Can you work these out from the model? Positions are in its coordinate system, mm. Face numbers are marked on the shaded views. A direction names the side the tool comes from. Give positions to 0.01 mm unless a question says otherwise; leave off trailing zeros. Order: outer loops, then holes, each group sorted by start corner. A loop starts at its lowest first (then second) coordinate and runs counter-clockwise, first axis right, second up. Notation, with made-up numbers: (82.5, 33.25) - (122.5, 33.25) arc R25 ccw to (122.5, 51.25) - close; hole circle Ø1 at (60.5, 37). An arc over 180 degrees is marked (long way). Answer as CSV lines item,"result".
```python
from build123d import *

# Parameters (mm, degrees)
SKETCH_1_W      = 120
SKETCH_1_H      = 150
EXTRUDE_1_DEPTH = 10
CHAMFER_1_SIZE  = 10
EXTRUDE_2_DEPTH = 20


with BuildPart() as part:
    # 草图1 → 凸台-拉伸1 (new, symmetric)
    with BuildSketch(Plane.XY):
        Rectangle(SKETCH_1_W, SKETCH_1_H)
    extrude(amount=EXTRUDE_1_DEPTH, both=True)

    # 倒角1
    chamfer_1_edges = [part.edges().sort_by_distance(p)[0] for p in [
        (-60, 75, 0),
        (60, 75, 0),
    ]]
    chamfer(chamfer_1_edges, length=CHAMFER_1_SIZE)

    # 草图2 → 凸台-拉伸2 (add)
    with BuildSketch(Plane(origin=(60, 0, 0), x_dir=(0, 0, -1), z_dir=(1, 0, 0))):
        Polygon((10, -75), (60, -75), (60, -65), (20, -15), (10, -15), align=None)
    extrude_2 = extrude(amount=-EXTRUDE_2_DEPTH)

    # 镜向1: 凸台-拉伸2 across plane
    add(extrude_2.mirror(Plane(origin=(0, 0, 0), x_dir=(0, 0, 1), z_dir=(1, 0, 0))))


solid = part.part
```
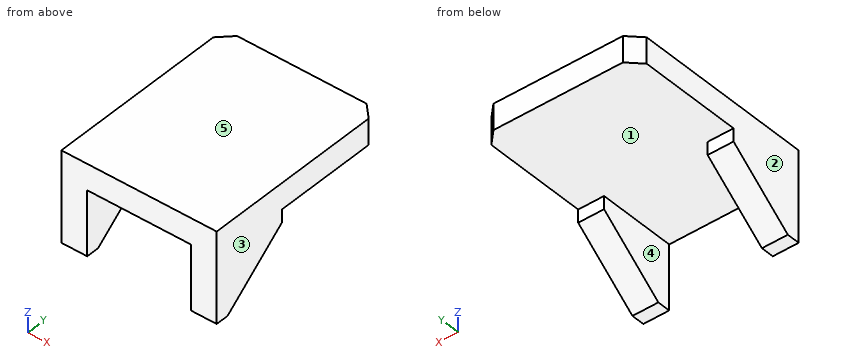
1) I'm going to push a flat-ended pin straight in: P1, Ø3, axis at x = -12.5, y = 14.5, coming from the -Z side. Where does the tip first touch, or does it pass through?
Answer block:
P1,"z = -10"
2) I want a section at B-B on x = -45. Write out the boundary of the cut face in (y, z), plus the area to 3 significant figures.
Answer block:
outline,"(-75, -60) - (-65, -60) - (-15, -20) - (-15, -10) - (75, -10) - (75, 10) - (-75, 10) - close"
area,"5,000 mm2"
3) If we mould it in two halves opening along X, with no side actions, what happens to the marked faces 1, 2 and 3? For each: +X half, -X half, draft (parallel to the pull), parting line (faces both ways), or undercut.
Answer block:
face 1,"undercut"
face 2,"-X half"
face 3,"+X half"
4) I want a section at A-A on z = -39. Write out the boundary of the cut face in (x, y), plus the area to 3 significant figures.
Answer block:
outline,"(-60, -75) - (-40, -75) - (-40, -38.75) - (-60, -38.75) - close; (40, -75) - (60, -75) - (60, -38.75) - (40, -38.75) - close"
area,"1,450 mm2"
5) I want a section at D-D on z = -15. Write out the boundary of the cut face in (x, y), plus the area to 3 significant figures.
Answer block:
outline,"(-60, -75) - (-40, -75) - (-40, -15) - (-60, -15) - close; (40, -75) - (60, -75) - (60, -15) - (40, -15) - close"
area,"2,400 mm2"
6) Which directions (+Z, -Z, +X, -X, +Y, -Y) give clear straight access to the entire face, cutting with the end or side of a thin tool? Please do the marked faces 4 and 5.
Answer block:
face 4,"-Z, +Y, -Y"
face 5,"+Z, +X, -X, +Y, -Y"
7) I want a section at C-C on y = -26. Write out the boundary of the cut face in (x, z).
Answer block:
outline,"(-60, -28.8) - (-40, -28.8) - (-40, -10) - (40, -10) - (40, -28.8) - (60, -28.8) - (60, 10) - (-60, 10) - close"
8) I need wall thicknesses on line 1 along X through (y, z) = (-62, -54); line 2 along Z through (x, y) = (9.5, 49.5); line 3 along Y through (x, z) = (-41, -18.5). Which ranges of each line are inside material? Lowest first, please. Write a range as [from, to].
Answer block:
line 1,"[-60, -40], [40, 60]"
line 2,"[-10, 10]"
line 3,"[-75, -15]"
